Input: part model. Units: mm. Frame: model coordinates. A direction names the side the tool comes from. Round coordinates to 2 decimals unless told otherwise and drop trailing zeros. Write each loop counter-clockwise with the first axis right and the second up, starting at its lowest first coordinate (ties: lowest second). Pieces come first, ordered by that corner, then holes. Notation, with made-up numbers: M -16,83.25 L 43,83.25 A15 ccw 43,88.25 Z; hole C -39,-20 d5. An arc over 180 degrees is marked long. Write each question's results on one line, items separated by ' | '. Start each with the question number.
```python
from build123d import *

# Parameters (mm, degrees)
SKETCH1_W           = 69.85
SKETCH1_H           = 12.7
BOSS_EXTRUDE1_DEPTH = 20.066
SKETCH3_R           = 7.62
CUT_EXTRUDE3_DEPTH  = 25.4
SKETCH4_R           = 1.27
CUT_EXTRUDE4_DEPTH  = 5.08


with BuildPart() as part:
    # Sketch1 → Boss-Extrude1 (new body)
    with BuildSketch(Plane(origin=(0, 0, 0), x_dir=(1, 0, 0), z_dir=(0, 1, 0))):
        Rectangle(SKETCH1_W, SKETCH1_H)
    extrude(amount=BOSS_EXTRUDE1_DEPTH)

    # Sketch3 → Cut-Extrude3 (cut)
    with BuildSketch(Plane(origin=(0, 0, -6.35), x_dir=(-1, 0, 0), z_dir=(0, 0, -1))):
        with Locations((0, 20.066)):
            Circle(SKETCH3_R)
    extrude(amount=-CUT_EXTRUDE3_DEPTH, mode=Mode.SUBTRACT)

    # Sketch4 → Cut-Extrude4 (cut)
    with BuildSketch(Plane(origin=(0, 0, 0), x_dir=(-1, 0, 0), z_dir=(0, -1, 0))):
        with Locations(Location((25.4, 0, 0), (0, 0, 90))):
            Circle(SKETCH4_R)
        with Locations(Location((-25.4, 0, 0), (0, 0, 90))):
            Circle(SKETCH4_R)
    extrude(amount=-CUT_EXTRUDE4_DEPTH, mode=Mode.SUBTRACT)


solid = part.part
```
1. Cut plane C-C on y = 15. Output: boundary loops of the cut face in (x, z) (3 decimals).
2. Contact query for a flat-ended pin moving along its axis: P1, Ø1.5, axis at x = 25.4, z = 0, coming from the -Y side. Output: stop coordinate, or through.
3. Cut plane D-D on z = 3.5. Output: boundary loops of the cut face in (x, y) (3 decimals).
4. Draft query along Z for faces 3 (the face through (-25, 5.08, 0)), 4 (the face through (34.925, 10, 0)), 5 (the face through (0, 10, -6.35)). Return one class per face: +Z half, -Z half, draft (parallel to the pull), parting line (faces both ways), or undercut.
5. Access query for faces 1 (the face through (-21, 20.066, 0)), 2 (the face through (25, 5.08, 0)). Directions: +Z, -Z, +X, -X, +Y, -Y. A direction counts if a zero-diameter tool reaches every point of the face in a straight line with its end or side. Return the directions, or none.
6. Cut plane B-B on x = 25.4. Output: boundary loops of the cut face in (y, z), and give its area (3 significant figures).
7. Cut plane A-A on z = 0. Output: boundary loops of the cut face in (x, y) (3 decimals), and give its area (3 significant figures).
8. Line query: L1, parallel to X at y = 1.95, z = 0 (3 decimals); L2, parallel to X at y = 15.75, z = -1 (3 decimals); L3, parallel to Y at x = 0, z = -5. Output: solid intervals per line, ascending. Write a range as from..to.
Answers follow:
1) outline: M -34.925,-6.35 L -5.692,-6.35 L -5.692,6.35 L -34.925,6.35 Z; M 5.692,-6.35 L 34.925,-6.35 L 34.925,6.35 L 5.692,6.35 Z
2) P1: stops at y = 5.08
3) outline: M -34.925,0 L 34.925,0 L 34.925,20.066 L 7.62,20.066 A7.62 cw -7.62,20.066 L -34.925,20.066 Z
4) face 3: undercut | face 4: draft | face 5: -Z half
5) face 1: +Z, -Z, +X, -X, +Y | face 2: -Y
6) outline: M 0,-6.35 L 20.07,-6.35 L 20.07,6.35 L 0,6.35 L 0,1.27 L 5.08,1.27 L 5.08,-1.27 L 0,-1.27 Z | area: 242 mm2
7) outline: M -34.925,0 L -26.67,0 L -26.67,5.08 L -24.13,5.08 L -24.13,0 L 24.13,0 L 24.13,5.08 L 26.67,5.08 L 26.67,0 L 34.925,0 L 34.925,20.066 L 7.62,20.066 A7.62 cw -7.62,20.066 L -34.925,20.066 Z | area: 1,280 mm2
8) L1: x = -34.925..-26.67, -24.13..24.13, 26.67..34.925 | L2: x = -34.925..-6.28, 6.28..34.925 | L3: y = 0..12.45
